CAD build for the part. Positions are in the model's coordinates, mm. A direction names the side the tool comes from. Give positions to 0.01 mm unless a question says otherwise; leave off trailing zeros. Loops run counter-clockwise (first coordinate to the right, second up) from the corner with the lowest first, then second, coordinate; pieces in that order, holes last. Notation, with made-up numbers: (83, 2) -> (127, 2) arc R17 cw to (127, 18) -> close; hole circle Ø8 at (44, 45). An arc over 180 degrees is marked (long way). Use one line per item in the form item = value.
Autodesk Inventor part; units mm, degrees
ref_plane "XZ Plane" through (0, 0, 0) normal (0, 1, 0) x (-1, 0, 0)
ref_plane "XY Plane" through (0, 0, 0) normal (0, 0, 1) x (1, 0, 0)
sketch "Sketch3" plane through (0, 0, 0) normal (0, 0, 1) x (1, 0, 0)
  line L0 (0, 0) -> (0, 127) construction
  line L1 (0, 0) -> (101.6, 0)
  line L2 (101.6, 0) -> (101.6, 203.2)
  line L3 (101.6, 203.2) -> (88.9, 203.2)
  line L4 (88.9, 203.2) -> (88.9, 12.7)
  line L5 (88.9, 12.7) -> (0, 12.7)
  line L6 (0, 12.7) -> (0, 0)
  dimension "d2" = 127
  dimension "forkWallThickness" = 12.7
  dimension "oneHalfTubeDiameter" = 88.9
  dimension "baseMaterialWidth" = 12.7
  dimension "d6" = 203.2
extrude "Extrusion1" add sketch "Sketch3" along normal mid plane 101.6
mirror "Mirror1" about plane through (0, 0, 0) normal (1, 0, 0) of "Extrusion1"
properties part number "forkV01"
1. Cut at B-B, the plane z = -28.5. Write the cut outline in (x, y).
Result sheet:
outline = (-101.6, 0) -> (101.6, 0) -> (101.6, 203.2) -> (88.9, 203.2) -> (88.9, 12.7) -> (-88.9, 12.7) -> (-88.9, 203.2) -> (-101.6, 203.2) -> close
2. Cut at A-A, the plane y = 158. Write the cut outline in (x, z), then the cut area to 3 significant figures.
Result sheet:
outline = (-101.6, -50.8) -> (-88.9, -50.8) -> (-88.9, 50.8) -> (-101.6, 50.8) -> close; (88.9, -50.8) -> (101.6, -50.8) -> (101.6, 50.8) -> (88.9, 50.8) -> close
area = 2,580 mm^2
3. Cut at C-C, the plane x = 45.5. Write the cut outline in (y, z).
Result sheet:
outline = (0, -50.8) -> (12.7, -50.8) -> (12.7, 50.8) -> (0, 50.8) -> close
4. Tool access for faces 1 (the flat face through (0, 12, -50.8)), 2 (the flat face through (-88.9, 107, -1)): list every direction of +Z, -Z, +X, -X, +Y, -Y with a clear straight run to the whole face (end or side of a thin tool).
Result sheet:
face_1 = -Z, +X, -X, +Y, -Y
face_2 = +Z, -Z, +Y
5. Drill centre lines: line 1 (X direction, y = 61, z = -11.5); line 2 (Y direction, x = -55, z = -39). Where is each one in solid material? Low to high.
Result sheet:
line_1 = -101.6 to -88.9, 88.9 to 101.6
line_2 = 0 to 12.7
6. Drop a flat-ended pin along its axis: P1, Ø4, axis at x = 16.5, z = 33.5, coming from the +Y side. Give the stop position or say it passes through.
Result sheet:
P1 = 12.7
